The model under review builds one solid part; all positions refer to its coordinate system, in mm. Face numbers are marked on the shaded views. A direction names the side the tool comes from. Coordinates: 2 decimals unless noted, no trailing zeros. Write each loop counter-clockwise with the first axis right and the second up, starting at its lowest first coordinate (ties: lowest second). Pieces come first, ordered by that corner, then holes. Notation, with made-up numbers: (-32.5, 31) - (8.5, 31) arc R24 ccw to (8.5, 67) - close; hole circle Ø3 at (4, 20). An arc over 180 degrees is marked (long way). Answer as CSV lines item,"result". Start each with the question number.
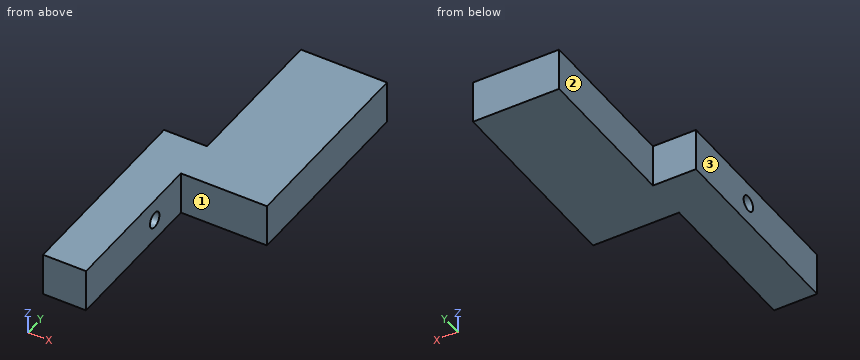
Autodesk Inventor part; units mm, degrees
ref_plane "YZ Plane" through (0, 0, 0) normal (1, 0, 0) x (0, 1, 0)
ref_plane "XZ Plane" through (0, 0, 0) normal (0, 1, 0) x (-1, 0, 0)
ref_plane "XY Plane" through (0, 0, 0) normal (0, 0, 1) x (1, 0, 0)
sketch "Sketch1" plane through (0, 0, 0) normal (0, 0, 1) x (1, 0, 0)
  line L0 (-8.0472, -28.1521) -> (1.9528, -28.1521)
  line L1 (1.9528, -28.1521) -> (1.9528, -64.3521)
  line L2 (1.9528, -64.3521) -> (-8.0472, -64.3521)
  line L3 (-8.0472, -64.3521) -> (-8.0472, -28.1521)
  point P0 (0, 0)
  dimension "d0" = 10
  dimension "d1" = 36.2
extrude "Extrusion1" add sketch "Sketch1" along normal blind 10
sketch "Sketch3" plane through (1.9528, -64.3521, 0) normal (1, 0, 0) x (0, 0, -1)
  line L0 (0, 36.2) -> (-10, 36.2)
  line L1 (-5, 36.2) -> (-5, 26.2)
  point P0 (0, 64.3521)
  dimension "d12" = 10
hole "Hole2" at (1.9528, -38.1521, 5) direction (-1, 0, 0) diameter 3.6 end through all
sketch "Sketch4" plane through (-8.0472, -28.1521, 0) normal (0, 1, 0) x (1, 0, 0)
  line L0 (10, -10) -> (0, -10)
  line L1 (10, 0) -> (10, -10)
  line L2 (0, -10) -> (10, -10)
  line L3 (10, -10) -> (10, 0)
  line L4 (10, 0) -> (0, 0)
  line L5 (0, 0) -> (0, -10)
  point P0 (8.0472, 0)
extrude "Extrusion2" add sketch "Sketch4" along normal blind 10
sketch "Sketch5" plane through (1.9528, -64.3521, 10) normal (1, 0, 0) x (0, 0, -1)
  line L0 (0, 0) -> (0, 46.2)
  line L1 (0, 46.2) -> (10, 46.2)
  line L2 (10, 46.2) -> (10, 36.2)
  line L3 (10, 36.2) -> (0, 36.2)
  line L4 (0, 36.2) -> (0, 46.2)
  point P0 (10, 64.3521)
  dimension "d22" = 10
  dimension "d23" = 10
extrude "Extrusion3" add sketch "Sketch5" along normal blind 20
sketch "Sketch6" plane through (-8.0472, -18.1521, 0) normal (0, 1, 0) x (1, 0, 0)
  line L0 (0, -10) -> (30, -10)
  line L1 (10, 0) -> (30, 0)
  line L2 (30, 0) -> (30, -10)
  line L3 (30, -10) -> (10, -10)
  line L4 (10, -10) -> (10, 0)
  point P0 (8.0472, 0)
  point P1 (10, -10)
extrude "Extrusion4" add sketch "Sketch6" along normal blind 50.8
sketch "Sketch7" plane through (-8.0472, 32.6479, 0) normal (0, 1, 0) x (1, 0, 0)
  line L0 (30, 0) -> (10, 0)
  line L1 (10, 0) -> (10, -10)
  line L2 (10, -10) -> (30, -10)
  line L3 (30, -10) -> (30, 0)
  point P0 (8.0472, 0)
extrude "Extrusion5" cut sketch "Sketch7" against normal blind 15
properties part number "lever staggered"
(1) Add section D-D on y = -59. Give the boundary of the cut face in (x, z), then the cut area to 3 significant figures.
(2) Add section A-A on z = 5. Give the boundary of the cut face in (x, y).
(3) Wall thickness on line 1 (Y direction, x = -2.75, z = 5); line 2 (X direction, y = -32, z = 9); line 3 (Y direction, x = 11.5, z = 4.5): over which ranges is each line inside the solid? List them lowest first.
(4) For pin 1 (8 mm diameter, centred on x = 8.5, y = 2.5, fed in from -Z); pin 2 (3 mm diameter, centred on y = -38.15, z = 5, fed in from -X), all flat-tipped, find the tip position at first contact; note any pin that passes through.
(5) Add section C-C on x = 17.75. Give the boundary of the cut face in (y, z), then the cut area to 3 significant figures.
(6) Add section B-B on z = 9.25. Give the boundary of the cut face in (x, y), then the cut area to 3 significant figures.
(7) For the marked faces 1, 2 and 3, list the 3-axis set-ups (+Z, -Z, +X, -X, +Y, -Y) from which the entire face can be reached by the end or side of a thin tool; tool diameter is ignored.
Reported:
1,outline,"(-8.05, 0) - (1.95, 0) - (1.95, 10) - (-8.05, 10) - close"
1,area,"100 mm²"
2,outline,"(-8.05, -64.35) - (1.95, -64.35) - (1.95, -39.95) - (-8.05, -39.95) - close; (-8.05, -36.35) - (1.95, -36.35) - (1.95, -28.15) - (21.95, -28.15) - (21.95, 17.65) - (1.95, 17.65) - (1.95, -18.15) - (-8.05, -18.15) - close"
3,line 1,"-64.35 to -39.95, -36.35 to -18.15"
3,line 2,"-8.05 to 1.95"
3,line 3,"-28.15 to 17.65"
4,pin 1,"z = 0"
4,pin 2,"through"
5,outline,"(-28.15, 0) - (17.65, 0) - (17.65, 10) - (-28.15, 10) - close"
5,area,"458 mm²"
6,outline,"(-8.05, -64.35) - (1.95, -64.35) - (1.95, -28.15) - (21.95, -28.15) - (21.95, 17.65) - (1.95, 17.65) - (1.95, -18.15) - (-8.05, -18.15) - close"
6,area,"1,380 mm²"
7,face 1,"+Z, -Z, +X, -Y"
7,face 2,"+Z, -Z, -X, +Y"
7,face 3,"+Z, -Z, -X, +Y, -Y"
